Read the model definition and answer for the solid it produces. Units are mm, in the model's axes. A direction names the side the tool comes from. Give positions to 0.01 mm unless a question says otherwise; leave off trailing zeros. Order: outer loops, then holes, each group sorted by start corner. A loop starts at its lowest first (then second) coordinate and runs counter-clockwise, first axis right, second up. Notation, with made-up numbers: (86, -2.5) - (120, -2.5) arc R25 cw to (120, 9.5) - close; hole circle Ø5 at (-14, 64). An arc over 180 degrees is marked (long way). Use a Markdown table: item, result. Add a question column.
1. A cutting plane is placed at B-B on z = 3.35. State how many separate pieces and enclosed holes the cut face has, and give its area (3 significant figures).
2. Consider L1, parallel to Y at x = -5, z = 1.95; L2, parallel to Y at x = 4, z = 1; L3, parallel to X at y = 21, z = 2.25. Determine where each line is inside the solid, lowest interval first.
3. For a pull along Y with two mould halves and no side action, classify faces 4 (the flat face through (-10, 17, 2)), 5 (the cylindrical face through (-5.195, 21.487, 1.972)), 6 (the flat face through (0, -25, 2)) as released by +Y, released by -Y, zero draft, split by the parting line, or undercut.
4. A cutting plane is placed at C-C on y = 0. Determine the outline of the cut face in (x, z), and give its area (3 significant figures).
5. A cutting plane is placed at D-D on x = -20. Determine the outline of the cut face in (y, z).
6. A cutting plane is placed at A-A on x = -5. Determine the outline of the cut face in (y, z), and give its area (3 significant figures).
7. Which of the six approach directions +Z, -Z, +X, -X, +Y, -Y give full straight-line access (tool end or side, diameter ignored) to faces 1 (the flat face through (-18, 10, 2)), 2 (the flat face through (-10, -18, 2)), 3 (the cylindrical face through (8.797, 23.859, 2.028))?
8. Flat-ended cylindrical pins translate along their axes: P1, Ø2.5, axis at x = -20, y = -5, coming from the -Z side; P2, Ø1.2, axis at y = -18.5, z = 3, coming from the -X side; P3, Ø2, axis at x = -16.5, z = 2, coming from the -Y side; P4, Ø2, axis at x = -14, z = 1.5, coming from the -Y side. Find the tip coordinate at first contact, or state that the pin passes through.
```python
from build123d import *

# Parameters (mm, degrees)
SKETCH_1_W      = 15
SKETCH_1_H      = 20
SKETCH_1_R      = 1.5
SKETCH_1_W_2    = 20
SKETCH_1_R_2    = 3.5
SKETCH_1_H_2    = 15
EXTRUDE_1_DEPTH = 4
FILLET_1_R      = 4


with BuildPart() as part:
    # 草图1 → 凸台-拉伸1 (new body)
    # profile 1 of 4: a face of its own
    with BuildSketch(Plane.XY):
        with Locations((-17.5, 0)):
            Rectangle(SKETCH_1_W, SKETCH_1_H)
        with Locations((-20, -5)):
            Circle(SKETCH_1_R, mode=Mode.SUBTRACT)
        with Locations((-20, 5)):
            Circle(SKETCH_1_R, mode=Mode.SUBTRACT)
    # profile 2 of 4: a face of its own
    with BuildSketch(Plane.XY):
        Rectangle(SKETCH_1_W_2, SKETCH_1_H)
        with Locations((-5, -5)):
            Circle(SKETCH_1_R, mode=Mode.SUBTRACT)
        Circle(SKETCH_1_R_2, mode=Mode.SUBTRACT)
        with Locations((5, -5)):
            Circle(SKETCH_1_R, mode=Mode.SUBTRACT)
        with Locations((-5, 5)):
            Circle(SKETCH_1_R, mode=Mode.SUBTRACT)
        with Locations((5, 5)):
            Circle(SKETCH_1_R, mode=Mode.SUBTRACT)
    # profile 3 of 4: a face of its own
    with BuildSketch(Plane.XY):
        with Locations((0, 17.5)):
            Rectangle(SKETCH_1_W_2, SKETCH_1_H_2)
        with Locations((-5, 20)):
            Circle(SKETCH_1_R, mode=Mode.SUBTRACT)
        with Locations((5, 20)):
            Circle(SKETCH_1_R, mode=Mode.SUBTRACT)
    # profile 4 of 4: a face of its own
    with BuildSketch(Plane.XY):
        with Locations((0, -17.5)):
            Rectangle(SKETCH_1_W_2, SKETCH_1_H_2)
        with Locations((-5, -20)):
            Circle(SKETCH_1_R, mode=Mode.SUBTRACT)
        with Locations((5, -20)):
            Circle(SKETCH_1_R, mode=Mode.SUBTRACT)
    extrude(amount=EXTRUDE_1_DEPTH)

    # 圆角1
    fillet_1_edges = [part.edges().sort_by_distance(p)[0] for p in [
        (-25, -10, 2),
        (-25, 10, 2),
        (-10, 10, 2),
        (-10, 25, 2),
        (10, 25, 2),
        (10, -25, 2),
        (-10, -25, 2),
        (-10, -10, 2),
    ]]
    fillet(fillet_1_edges, radius=FILLET_1_R)


solid = part.part
```
Output values:
| question | item | result |
|---|---|---|
| 1 | separate pieces | 1 |
| 1 | enclosed holes | 11 |
| 1 | area | 1,180 mm² |
| 2 | L1 | -25 to -21.5, -18.5 to -6.5, -3.5 to 3.5, 6.5 to 18.5, 21.5 to 25 |
| 2 | L2 | -25 to -21.12, -18.88 to -6.12, -3.88 to 3.88, 6.12 to 18.88, 21.12 to 25 |
| 2 | L3 | -10 to -6.12, -3.88 to 3.88, 6.12 to 10 |
| 3 | face 4 | zero draft |
| 3 | face 5 | undercut |
| 3 | face 6 | released by -Y |
| 4 | outline | (-25, 0) - (-3.5, 0) - (-3.5, 4) - (-25, 4) - close; (3.5, 0) - (10, 0) - (10, 4) - (3.5, 4) - close |
| 4 | area | 112 mm² |
| 5 | outline | (-10, 0) - (-6.5, 0) - (-6.5, 4) - (-10, 4) - close; (-3.5, 0) - (3.5, 0) - (3.5, 4) - (-3.5, 4) - close; (6.5, 0) - (10, 0) - (10, 4) - (6.5, 4) - close |
| 6 | outline | (-25, 0) - (-21.5, 0) - (-21.5, 4) - (-25, 4) - close; (-18.5, 0) - (-6.5, 0) - (-6.5, 4) - (-18.5, 4) - close; (-3.5, 0) - (3.5, 0) - (3.5, 4) - (-3.5, 4) - close; (6.5, 0) - (18.5, 0) - (18.5, 4) - (6.5, 4) - close; (21.5, 0) - (25, 0) - (25, 4) - (21.5, 4) - close |
| 6 | area | 152 mm² |
| 7 | face 1 | +Z, -Z, -X, +Y |
| 7 | face 2 | +Z, -Z, -X, -Y |
| 7 | face 3 | +Z, -Z, +X, +Y |
| 8 | P1 | through |
| 8 | P2 | x = -10 |
| 8 | P3 | y = -10 |
| 8 | P4 | y = -10.13 |
